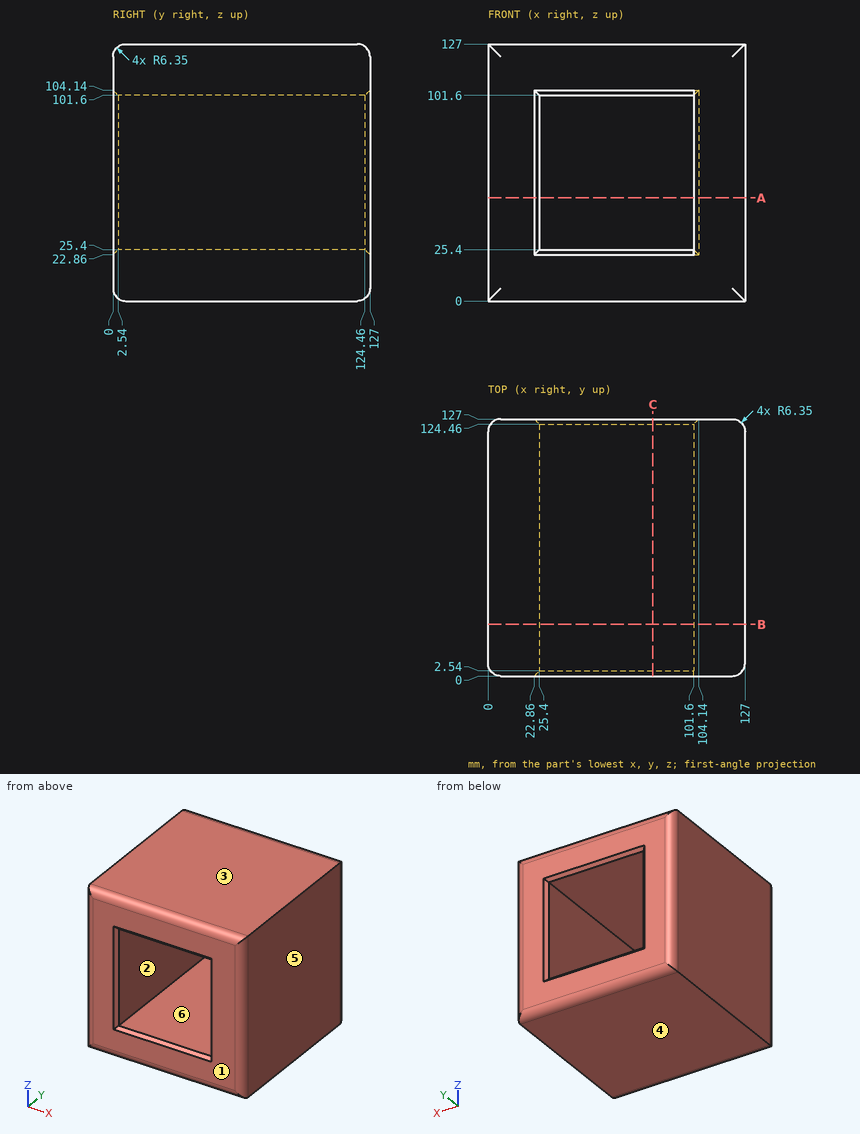
Drawing for the job (mm, zero at the part's lowest x, y, z). A direction names the side the tool comes from. Give positions to 0.01 mm unless a question says otherwise; leave off trailing zeros. Loops run counter-clockwise (first coordinate to the right, second up) from the corner with the lowest first, then second, coordinate; pieces in that order, holes last.
1) 3-axis set-ups, long thin cutter, end or side, ignore diameter. For the marked faces 5 and 6: which of +Z, -Z, +X, -X, +Y, -Y reach the whole face in a straight line?
Values follow:
face 5: +Z, -Z, +X, +Y, -Y
face 6: +Y, -Y
2) Two-plate mould, pull along Z, no slides. Class the marked faces 1, 2, 3 and 4: released by +Z, released by -Z, zero draft, split by the parting line, or undercut.
Values follow:
face 1: zero draft
face 2: undercut
face 3: released by +Z
face 4: released by -Z
3) Band-saw the part on B-B on y = 25.5. List the corners of the cut face in (x, z), then the cut area to 3 significant figures.
Values follow:
outline: (0, 0) - (127, 0) - (127, 127) - (0, 127) - close; hole (25.4, 25.4) - (101.6, 25.4) - (101.6, 101.6) - (25.4, 101.6) - close
area: 10,300 mm2
4) Probe line 1 along X through (y, z) = (105, 98.5); line 2 along Y through (x, z) = (103, 23.5). List the from-to ranges inside material, lowest first.
Values follow:
line 1: x = 0 to 25.4, 101.6 to 127
line 2: y = 0 to 126.36
5) Band-saw the part on C-C on x = 81.5. List the corners of the cut face in (y, z), then the cut area to 3 significant figures.
Values follow:
outline: (0, 6.35) arc R6.35 ccw to (6.35, 0) - (120.65, 0) arc R6.35 ccw to (127, 6.35) - (127, 22.86) - (124.46, 25.4) - (2.54, 25.4) - (0, 22.86) - close; (0, 104.14) - (2.54, 101.6) - (124.46, 101.6) - (127, 104.14) - (127, 120.65) arc R6.35 ccw to (120.65, 127) - (6.35, 127) arc R6.35 ccw to (0, 120.65) - close
area: 6,400 mm2
6) Band-saw the part on A-A on z = 51. List the corners of the cut face in (x, y), then the cut area to 3 significant figures.
Values follow:
outline: (0, 6.35) arc R6.35 ccw to (6.35, 0) - (22.86, 0) - (25.4, 2.54) - (25.4, 124.46) - (22.86, 127) - (6.35, 127) arc R6.35 ccw to (0, 120.65) - close; (101.6, 0) - (120.65, 0) arc R6.35 ccw to (127, 6.35) - (127, 120.65) arc R6.35 ccw to (120.65, 127) - (104.14, 127) - (101.6, 124.46) - close
area: 6,410 mm2
